The drawing under review shows one solid part. Ordinate dimensions are in mm from its lowest x, y, z. A direction names the side the tool comes from. Give positions to 0.01 mm unless a question says otherwise; leave off trailing zeros. Order: outer loops, then holes, each group sorted by start corner. A loop starts at its lowest first (then second) coordinate and runs counter-clockwise, first axis right, second up. Notation, with made-up numbers: (-5.75, 19.25) -> (23.25, 19.25) arc R32 ccw to (23.25, 50.25) -> close; hole circle Ø4 at (2.5, 50). An arc over 180 degrees is marked (long way). One line per item, written item: value.
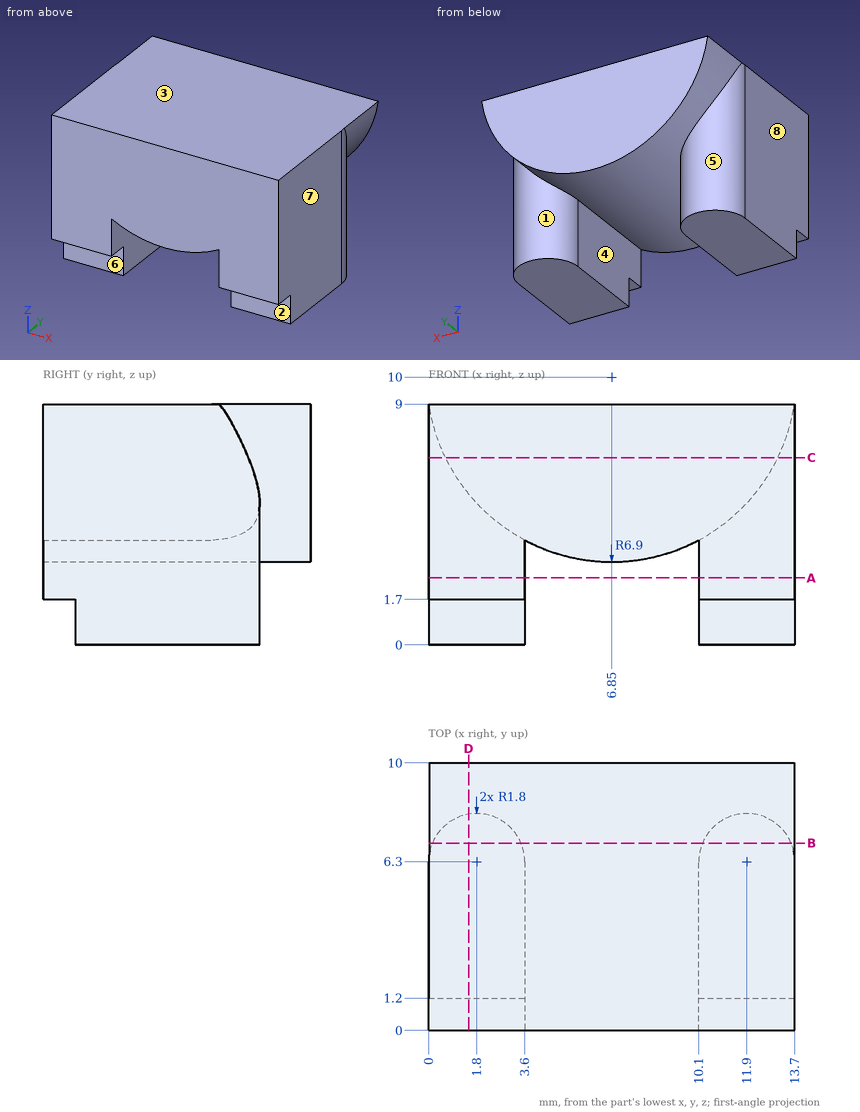
Item 1: Draft analysis for pull direction X (two halves, no side actions). For the marked faces 5, 6, 7 and 8, state which applies: pulls with the +X half, pulls with the -X half, needs draft (parallel to the pull), parting line crosses it, or undercut.
Returned:
face 5: undercut
face 6: needs draft
face 7: pulls with the +X half
face 8: pulls with the -X half
Item 2: Machinability: for the marked faces 1, 2, 3 and 4, which of the approach directions +Z, -Z, +X, -X, +Y, -Y give a long, thin tool a straight path to every point of the face, cutting with its end or side? Answer none if there is none.
Returned:
face 1: -Z, +Y
face 2: -Z, +X, -X, -Y
face 3: +Z, +X, -X, +Y, -Y
face 4: -Z, +Y, -Y
Item 3: Add section A-A on z = 2.5. Give the boundary of the cut face in (x, y), plus the area to 3 significant figures.
Returned:
outline: (0, 0) -> (3.6, 0) -> (3.6, 6.3) arc R1.8 ccw to (0, 6.3) -> close; (10.1, 0) -> (13.7, 0) -> (13.7, 6.3) arc R1.8 ccw to (10.1, 6.3) -> close
area: 55.5 mm²
Item 4: To check wall thickness, follow line 1 along X through (y, z) = (4, 1); line 2 along Z through (x, y) = (13.25, 1); line 3 along Z through (x, y) = (5, 7.5). State the ranges of each line that lie inside material, in increasing order. Write a range as from..to.
Returned:
line 1: 0..3.6, 10.1..13.7
line 2: 1.7..9
line 3: 3.35..9
Item 5: Add section C-C on z = 7. Give the boundary of the cut face in (x, y).
Returned:
outline: (0, 0) -> (13.7, 0) -> (13.7, 6.3) arc R1.8 ccw to (13.06, 7.67) -> (13.06, 10) -> (0.64, 10) -> (0.64, 7.67) arc R1.8 ccw to (0, 6.3) -> close
Item 6: Add section D-D on x = 1.5. Give the boundary of the cut face in (y, z), plus the area to 3 significant figures.
Returned:
outline: (0, 1.7) -> (1.2, 1.7) -> (1.2, 0) -> (8.07, 0) -> (8.07, 5.64) -> (10, 5.64) -> (10, 9) -> (0, 9) -> close
area: 77.1 mm²
Item 7: Clearance check with flat-ended pins moving along their axes: P1, Ø1, axis at x = 12.5, y = 0.5, coming from the -Z side; P2, Ø0.5, axis at x = 1.5, z = 1, coming from the -Y side; P3, Ø1, axis at x = 4.5, y = 3, coming from the -Z side. State where each tip first meets the part, or that it passes through.
Returned:
P1: z = 1.7
P2: y = 1.2
P3: z = 3.35
Item 8: Add section B-B on y = 7. Give the boundary of the cut face in (x, z), plus the area to 3 significant figures.
Returned:
outline: (0.02, 9) arc R6.9 ccw to (0.14, 8.38) -> (0.14, 0) -> (3.46, 0) -> (3.46, 3.99) arc R6.9 ccw to (10.24, 3.99) -> (10.24, 0) -> (13.56, 0) -> (13.56, 8.38) arc R6.9 ccw to (13.68, 9) -> close
area: 97.8 mm²
